Check sheet for the drawn part. Datum: minimum x, y, z corner. Units: mm. Coordinates: 2 decimals unless noted, no trailing zeros. Write each loop counter-clockwise with the first axis right and the second up, starting at its lowest first coordinate (ties: lowest second). Pieces come first, ordered by that corner, then holes. Notation, with made-up numbers: (88.25, 11.5) -> (130.25, 11.5) arc R4 ccw to (130.25, 18.5) -> close; hole circle Ø2 at (6.25, -16.5). An arc over 180 degrees is marked (long way). Answer in a Markdown table with one row per item. Add a question column.
Q1. Gauge pin test, flat ends, axial feed: P1, Ø3, axis at y = 6.5, z = 3, coming from the +X side; P2, Ø3, axis at x = 83, z = 38, coming from the -Y side; P3, Ø4, axis at y = 21.5, z = 79, coming from the -X side. Record the tip position at first contact, or that the pin passes through.
Q2. Release check for a two-part mould opening along Z. For the marked faces 1, 2, 3 and 4 record: pulls with the +Z half, pulls with the -Z half, needs draft (parallel to the pull), parting line crosses it, or undercut.
Q3. Section check D-D, the plane z = 13. Record the boundary of the cut face in (x, y), and give its area (3 significant figures).
Q4. Section check A-A, the plane x = 140. Record the boundary of the cut face in (y, z).
Q5. Section check B-B, the plane y = 15. Record the boundary of the cut face in (x, z), and give its area (3 significant figures).
Q6. Thickness scan on line 1 (Z direction, x = 93, y = 13.25); line 2 (Y direction, x = 36.5, z = 18); line 3 (Y direction, x = 35, z = 173.45). Record the ranges inside material, lowest first.
Q7. Section check C-C, the plane x = 104. Record the boundary of the cut face in (y, z), and give its area (3 significant figures).
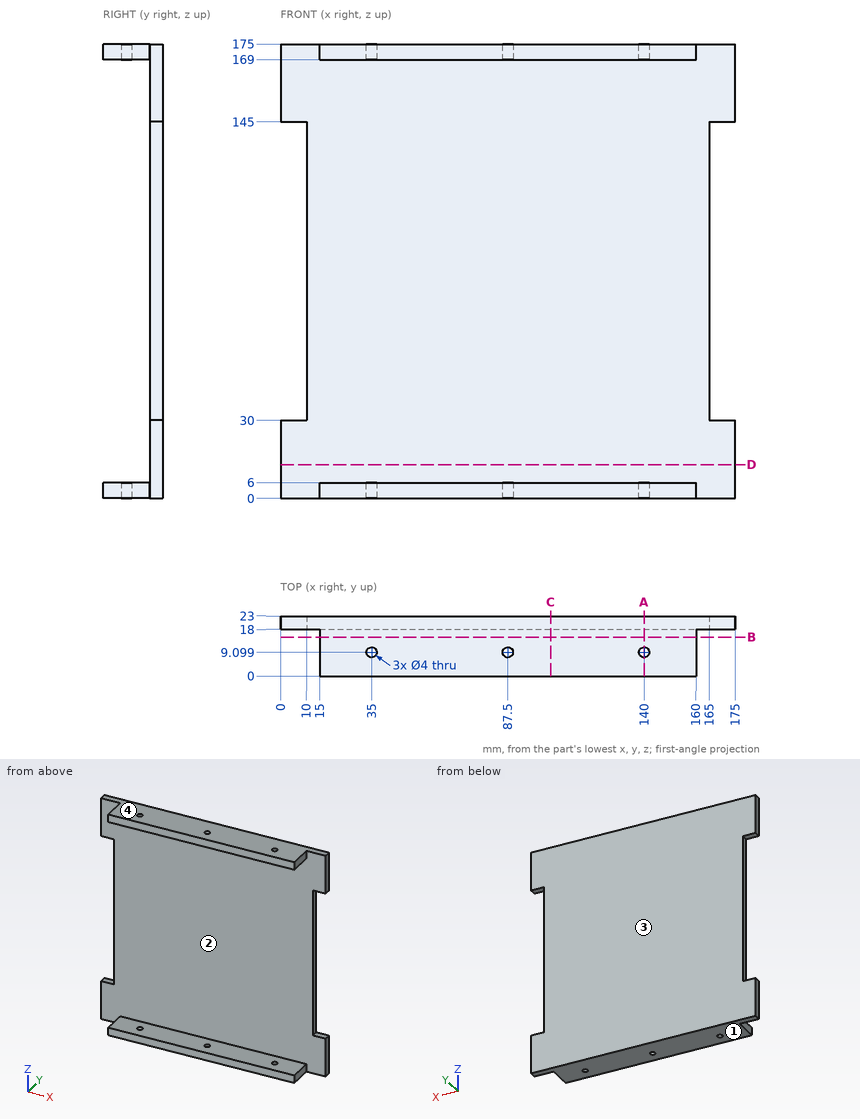
Calculated:
| question | item | result |
|---|---|---|
| 1 | P1 | stops at x = 160 |
| 1 | P2 | stops at y = 18 |
| 1 | P3 | stops at x = 10 |
| 2 | face 1 | pulls with the -Z half |
| 2 | face 2 | undercut |
| 2 | face 3 | needs draft |
| 2 | face 4 | pulls with the +Z half |
| 3 | outline | (0, 18) -> (175, 18) -> (175, 23) -> (0, 23) -> close |
| 3 | area | 875 mm² |
| 4 | outline | (0, 0) -> (7.1, 0) -> (7.1, 6) -> (0, 6) -> close; (0, 169) -> (7.1, 169) -> (7.1, 175) -> (0, 175) -> close; (11.1, 0) -> (23, 0) -> (23, 175) -> (11.1, 175) -> (11.1, 169) -> (18, 169) -> (18, 6) -> (11.1, 6) -> close |
| 5 | outline | (15, 0) -> (160, 0) -> (160, 6) -> (15, 6) -> close; (15, 169) -> (160, 169) -> (160, 175) -> (15, 175) -> close |
| 5 | area | 1,740 mm² |
| 6 | line 1 | z = 0 to 6, 169 to 175 |
| 6 | line 2 | y = 18 to 23 |
| 6 | line 3 | y = 0 to 7.1, 11.1 to 23 |
| 7 | outline | (0, 0) -> (23, 0) -> (23, 175) -> (0, 175) -> (0, 169) -> (18, 169) -> (18, 6) -> (0, 6) -> close |
| 7 | area | 1,090 mm² |
